Here's how the part is built. I have some questions about the finished solid (model axes, mm). Face numbers are marked on the shaded views. A direction names the side the tool comes from. Give positions to 0.01 mm unless a question says otherwise; leave off trailing zeros. Order: outer loops, then holes, each group sorted by start corner. A loop starts at its lowest first (then second) coordinate and runs counter-clockwise, first axis right, second up. Notation, with made-up numbers: M -29.5,88 L 4.5,88 A17 ccw 4.5,121 Z; hole C -7,-12.5 d1. An arc over 180 degrees is marked long. One line per item, written item: value. Start each with the question number.
from build123d import *

# Parameters (mm, degrees)
FILLET1_R     = 2.5
CHAMFER2_SIZE = 1


with BuildPart() as part:
    # Sketch1 → Revolve1 (revolve)
    with BuildSketch(Plane.XY, mode=Mode.PRIVATE) as revolve1_sk:
        Polygon((0, 0), (0, 12.5), (40, 12.5), (45, 17.5), (55, 17.5), (55, 15), (91, 15), (91, 12.5), (131, 12.5), (131, 0), align=None)
    revolve(revolve1_sk.sketch.rotate(Axis((131, 0, 0), (-1, 0, 0)), 90), axis=Axis((131, 0, 0), (-1, 0, 0)))

    # Fillet1
    fillet1_edges = [part.edges().sort_by_distance(p)[0] for p in [
        (91, 0, 12.5),
        (55, 0, 15),
    ]]
    fillet(fillet1_edges, radius=FILLET1_R - 0.0001)  # a hair under: the kernel refuses the full size

    # Chamfer2
    chamfer2_edges = [part.edges().sort_by_distance(p)[0] for p in [
        (0, 0, 12.5),
        (131, 0, 12.5),
    ]]
    chamfer(chamfer2_edges, length=CHAMFER2_SIZE)


solid = part.part
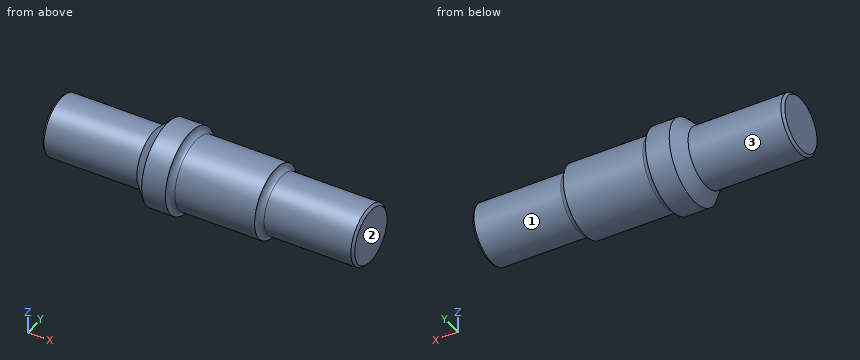
Item 1: I want a section at D-D on x = 84.5. Write out the boundary of the cut face in (y, z), plus the area to 3 significant figures.
Item 2: For the marked faces 1, 2 and 3, which set-ups out of +Z, -Z, +X, -X, +Y, -Y let a thin tool reach every point of the face, with its end or its side?
Item 3: Will these pins go through, and if not, where does the flat tip stop? P1, Ø3, axis at x = 111, y = -8, coming from the -Z side; P2, Ø3, axis at x = 72.5, z = -11, coming from the -Y side; P3, Ø4, axis at x = 76.5, z = -0.5, coming from the -Y side.
Item 4: I want a section at C-C on x = 37. Write out the boundary of the cut face in (y, z), plus the area to 3 significant figures.
Item 5: Please list where these lines run through material, in increasing order: probe 1 along Y at (x, z) = (82, 3); probe 2 along Z at (x, y) = (60, 5); probe 3 along Z at (x, y) = (22, -7). Write a range as [from, to].
Answer below:
1. outline: C 0,0 d30
1. area: 707 mm²
2. face 1: +X
2. face 2: +Z, -Z, +X, +Y, -Y
2. face 3: -X
3. P1: stops at z = -10.68
3. P2: stops at y = -11.61
3. P3: stops at y = -15
4. outline: C 0,0 d25
4. area: 491 mm²
5. probe 1: y = [-14.7, 14.7]
5. probe 2: z = [-14.14, 14.14]
5. probe 3: z = [-10.36, 10.36]
